Build history of the part. All positions in model axes, mm. Face numbers are marked on the shaded views. A direction names the side the tool comes from. Round coordinates to 2 decimals unless told otherwise and drop trailing zeros. Write each loop counter-clockwise with the first axis right and the second up, starting at its lowest first coordinate (ties: lowest second). Pieces come first, ordered by that corner, then holes.
Item 1: Drop flat-ended pins along their axis: pin 1 Ø3 at (x, y) = (19.6, 5) entering from +Z; pin 2 Ø6 at (x, y) = (33, -2.5) entering from +Z; pin 3 Ø2 at (y, z) = (5, -3) entering from -X; pin 4 Ø4 at (y, z) = (2.5, -17.5) entering from +X. Give the stop position or say it passes through.
Item 2: Band-saw the part on A-A, the plane y = -4. Write the cut outline in (x, z), then the cut area to 3 significant figures.
Item 3: Band-saw the part on D-D, the plane x = 5. Write the cut outline in (y, z).
Item 4: Wall check: probe 1 along Z at (x, y) = (11.6, 6.25); probe 2 along X at (y, z) = (-4, -13); probe 3 along X at (y, z) = (9, -8.5). Give the ranges that are in metal, low to high.
Item 5: Band-saw the part on C-C, the plane y = 5. Count the separate pieces of the cut face and the enclosed holes in it, then the cut area to 3 significant figures.
Item 6: Mould opens along X. For the marked faces 1, 2, 3 and 4 say: +X half, -X half, draft (parallel to the pull), parting line (faces both ways), or undercut.
Item 7: 3-axis set-ups, long thin cutter, end or side, ignore diameter. For the marked faces 5 and 6: which of +Z, -Z, +X, -X, +Y, -Y reach the whole face in a straight line?
Item 8: Band-saw the part on B-B, the plane z = -7.25. Write the cut outline in (x, y).
```python
from build123d import *

# Parameters (mm, degrees)
SKETCH1_W                      = 39.2
SKETCH1_H                      = 25
BOSS_EXTRUDE1_DEPTH            = 10
F_3_5_3_5_DIAMETER_HOLE1_D     = 3.5
SKETCH9_W                      = 14.6
SKETCH9_H                      = 25
BOSS_EXTRUDE2_DEPTH            = 10.5
SKETCH10_W                     = 5.65
SKETCH10_H                     = 2.55
CUT_EXTRUDE4_DEPTH             = 10
F_2_5_2_5_DIAMETER_HOLE1_D     = 2.5
F_2_5_2_5_DIAMETER_HOLE1_DEPTH = 7
F_2_5_2_5_DIAMETER_HOLE1_TIP   = 0.751075774
F_3_4_3_4_DIAMETER_HOLE1_D     = 3.4
CHAMFER1_SIZE                  = 10
FILLET5_R                      = 4.5
FILLET6_R                      = 1.5
F_3_4_3_4_DIAMETER_HOLE2_D     = 3.4
F_3_4_3_4_DIAMETER_HOLE2_DEPTH = 4
F_3_4_3_4_DIAMETER_HOLE2_TIP   = 1.021463052


with BuildPart() as part:
    # Sketch1 → Boss-Extrude1 (new body)
    with BuildSketch(Plane(origin=(0, 0, 0), x_dir=(1, 0, 0), z_dir=(0, 1, 0))):
        with Locations((19.6, 12.5)):
            Rectangle(SKETCH1_W, SKETCH1_H)
    extrude(amount=BOSS_EXTRUDE1_DEPTH)

    # Ø3.5 (3.5) Diameter Hole1 (through all)
    with Locations(Plane(origin=(0, 0, -25), x_dir=(-1, 0, 0), z_dir=(0, 0, -1))):
        with Locations((-19.6, 5)):
            Hole(F_3_5_3_5_DIAMETER_HOLE1_D / 2)

    # Sketch9 → Boss-Extrude2 (add)
    with BuildSketch(Plane.XZ):
        with Locations((31.9, -12.5)):
            Rectangle(SKETCH9_W, SKETCH9_H)
        with Locations((7.3, -12.5)):
            Rectangle(SKETCH9_W, SKETCH9_H)
    extrude(amount=BOSS_EXTRUDE2_DEPTH)

    # Sketch10 → Cut-Extrude4 (cut)
    with BuildSketch(Plane(origin=(0, 10, 0), x_dir=(1, 0, 0), z_dir=(0, 1, 0))):
        with Locations((19.6, 12.995)):
            Rectangle(SKETCH10_W, SKETCH10_H)
    extrude(amount=-CUT_EXTRUDE4_DEPTH, mode=Mode.SUBTRACT)

    # Ø2.5 (2.5) Diameter Hole1
    with Locations(Plane(origin=(0, 10, 0), x_dir=(1, 0, 0), z_dir=(0, 1, 0))):
        with Locations((11.6, 3), (27.6, 3), (27.6, 9.5), (11.6, 9.5)):
            Hole(F_2_5_2_5_DIAMETER_HOLE1_D / 2, depth=F_2_5_2_5_DIAMETER_HOLE1_DEPTH)
            with Locations((0, 0, -(F_2_5_2_5_DIAMETER_HOLE1_DEPTH + F_2_5_2_5_DIAMETER_HOLE1_TIP / 2))):  # 118° drill point
                Cone(0, F_2_5_2_5_DIAMETER_HOLE1_D / 2, F_2_5_2_5_DIAMETER_HOLE1_TIP, mode=Mode.SUBTRACT)

    # Ø3.4 (3.4) Diameter Hole1 (through all)
    with Locations(Plane(origin=(0, 10, 0), x_dir=(1, 0, 0), z_dir=(0, 1, 0))):
        with Locations((34.2, 13), (5, 13)):
            Hole(F_3_4_3_4_DIAMETER_HOLE1_D / 2)

    # Chamfer1
    chamfer1_edges = [part.edges().sort_by_distance(p)[0] for p in [
        (0, -0.25, 0),
        (0, -0.25, -25),
        (39.2, -0.25, -25),
        (39.2, -0.25, 0),
    ]]
    chamfer(chamfer1_edges, length=CHAMFER1_SIZE)

    # Fillet5
    fillet5_edges = [part.edges().sort_by_distance(p)[0] for p in [
        (39.2, -0.25, -10),
        (0, -0.25, -10),
        (0, -0.25, -15),
        (29.2, -0.25, -25),
        (10, -0.25, -25),
        (29.2, -0.25, 0),
        (10, -0.25, 0),
        (39.2, -0.25, -15),
    ]]
    fillet(fillet5_edges, radius=FILLET5_R)

    # Fillet6
    fillet6_edges = [part.edges().sort_by_distance(p)[0] for p in [
        (19.6, 0, 0),
    ]]
    fillet(fillet6_edges, radius=FILLET6_R)

    # Ø3.4 (3.4) Diameter Hole2
    with Locations(Plane(origin=(0, -10.5, 0), x_dir=(-1, 0, 0), z_dir=(0, -1, 0))):
        with Locations((-9.6, 13), (-29.6, 13)):
            Hole(F_3_4_3_4_DIAMETER_HOLE2_D / 2, depth=F_3_4_3_4_DIAMETER_HOLE2_DEPTH)
            with Locations((0, 0, -(F_3_4_3_4_DIAMETER_HOLE2_DEPTH + F_3_4_3_4_DIAMETER_HOLE2_TIP / 2))):  # 118° drill point
                Cone(0, F_3_4_3_4_DIAMETER_HOLE2_D / 2, F_3_4_3_4_DIAMETER_HOLE2_TIP, mode=Mode.SUBTRACT)


solid = part.part
```
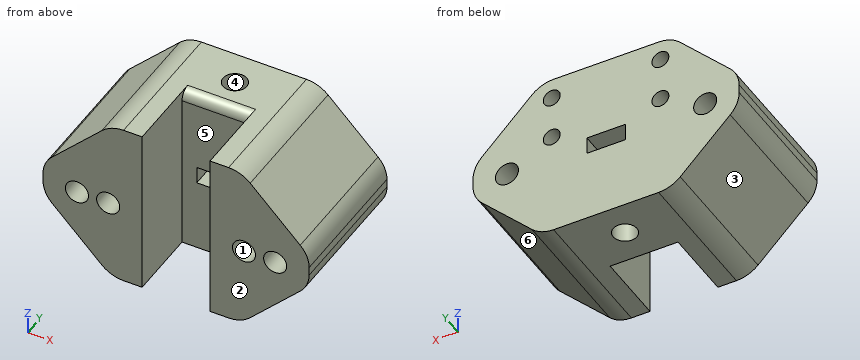
Results:
1. pin 1: passes through
1. pin 2: stops at z = -0.87
1. pin 3: stops at x = 6
1. pin 4: stops at x = 38.53
2. outline: (0, -13.14) arc R4.5 ccw to (1.32, -16.32) - (8.68, -23.68) arc R4.5 ccw to (11.86, -25) - (14.6, -25) - (14.6, 0) - (11.86, 0) arc R4.5 ccw to (8.68, -1.32) - (1.32, -8.68) arc R4.5 ccw to (0, -11.86) - close; (24.6, -25) - (27.34, -25) arc R4.5 ccw to (30.52, -23.68) - (37.88, -16.32) arc R4.5 ccw to (39.2, -13.14) - (39.2, -11.86) arc R4.5 ccw to (37.88, -8.68) - (30.52, -1.32) arc R4.5 ccw to (27.34, 0) - (24.6, 0) - close; hole circle Ø3.4 at (5, -13); hole circle Ø3.4 at (34.2, -13)
2. area: 508 mm2
3. outline: (-10.5, -20) - (10, -20) - (10, -14.7) - (-10.5, -14.7) - close; (-10.5, -11.3) - (10, -11.3) - (10, -5) - (-10.5, -5) - close
4. probe 1: z = -24.99 to -10.75, -8.25 to -4.25, -1.75 to -0.01
4. probe 2: x = 0 to 3.3, 6.7 to 14.6, 24.6 to 32.5, 35.9 to 39.2
4. probe 3: x = 1.5 to 10.85, 12.35 to 26.85, 28.35 to 37.7
5. separate pieces: 2
5. enclosed holes: 6
5. area: 646 mm2
6. face 1: undercut
6. face 2: draft
6. face 3: -X half
6. face 4: undercut
7. face 5: +Z, -Z, -Y
7. face 6: -Z, +X, +Y, -Y
8. outline: (2.75, -10.5) - (14.6, -10.5) - (14.6, 0) - (24.6, 0) - (24.6, -10.5) - (36.45, -10.5) - (36.45, 10) - (2.75, 10) - close; hole circle Ø3.5 at (19.6, 5)
